The model under review builds one solid part; all positions refer to its coordinate system, in mm. A direction names the side the tool comes from. Give positions to 0.01 mm unless a question says otherwise; leave off trailing zeros. Order: outer loops, then holes, each group sorted by start corner. A loop starts at its lowest first (then second) coordinate and runs counter-clockwise, first axis right, second up. Notation, with made-up numbers: (-23.75, -10) -> (-3.75, -10) arc R21 ccw to (-3.75, 26) -> close; hole circle Ø7 at (-4, 87.25). An arc over 180 degrees is marked (long way). Use one line per item in the form item = value.
```python
from build123d import *

# Parameters (mm, degrees)
SKETCH_W     = 30
SKETCH_H     = 30
PAD_DEPTH    = 2
SKETCH001_W  = 3
SKETCH001_H  = 26
PAD001_DEPTH = 4
SKETCH002_W  = 30
SKETCH002_H  = 2
PAD002_DEPTH = 5
SKETCH003_R  = 1
SKETCH003_W  = 9
SKETCH003_H  = 5
POCKET_DEPTH = 10


with BuildPart() as part:
    # Sketch → Pad (new body)
    with BuildSketch(Plane.XY):
        Rectangle(SKETCH_W, SKETCH_H)
    extrude(amount=PAD_DEPTH)

    # Sketch001 (on Face6 of Pad) → Pad001 (join)
    with BuildSketch(Plane.XY.offset(2)):
        with Locations((-13.5, 0)):
            Rectangle(SKETCH001_W, SKETCH001_H)
        with Locations((13.5, 0)):
            Rectangle(SKETCH001_W, SKETCH001_H)
    extrude(amount=PAD001_DEPTH)

    # Sketch002 (on Face5 of Pad001) → Pad002 (join)
    with BuildSketch(Plane.XY.offset(2)):
        with Locations((0, -14)):
            Rectangle(SKETCH002_W, SKETCH002_H)
        with Locations((0, 14)):
            Rectangle(SKETCH002_W, SKETCH002_H)
    extrude(amount=PAD002_DEPTH)

    # Sketch003 (on Face16 of Pad002) → Pocket (cut)
    with BuildSketch(Plane.XY.offset(7)):
        with Locations((-12.5, 12.5)):
            Circle(SKETCH003_R)
        with Locations((-12.5, -12.5)):
            Circle(SKETCH003_R)
        with Locations((12.5, -12.5)):
            Circle(SKETCH003_R)
        with Locations((12.5, 12.5)):
            Circle(SKETCH003_R)
        with Locations((4.5, -12.5)):
            Rectangle(SKETCH003_W, SKETCH003_H)
    extrude(amount=-POCKET_DEPTH, mode=Mode.SUBTRACT)


solid = part.part
```
1. The part is to be moulded in two halves that separate along X. For faces 4 (the face through (-15, 0, 3)), 5 (the face through (13, 0, 6)), 6 (the face through (9, -14, 3)), say which applies: +X half, -X half, draft (parallel to the pull), parting line (faces both ways), or undercut.
Values:
face_4 = -X half
face_5 = draft
face_6 = undercut
2. Add section D-D on y = -4. Give the boundary of the cut face in (x, z), then the cut area to 3 significant figures.
Values:
outline = (-15, 0) -> (15, 0) -> (15, 6) -> (12, 6) -> (12, 2) -> (-12, 2) -> (-12, 6) -> (-15, 6) -> close
area = 84.0 mm^2
3. Add section B-B on y = 12.5. Give the boundary of the cut face in (x, z), then the cut area to 3 significant figures.
Values:
outline = (-15, 0) -> (-13.5, 0) -> (-13.5, 6) -> (-15, 6) -> close; (-11.5, 0) -> (11.5, 0) -> (11.5, 2) -> (-11.5, 2) -> close; (13.5, 0) -> (15, 0) -> (15, 6) -> (13.5, 6) -> close
area = 64.0 mm^2
4. Tool access review of faces 1 (the face through (14.2, -13, 6.5)), 2 (the face through (0, -14, 3)), 3 (the face through (12, 0, 4)): name each direction out of +Z, -Z, +X, -X, +Y, -Y from which nothing blocks a thin tool from reaching the whole face with its end or side.
Values:
face_1 = +Z, +X, -X
face_2 = +Z, -Z, -Y
face_3 = +Z
5. For pin 1 Ø0.9 at (x, y) = (-13.5, -4.5) entering from +Z; pin 2 Ø1.6 at (x, z) = (2.5, 1) entering from -Y, all flat-tipped, find the tip position at first contact; note any pin that passes through.
Values:
pin_1 = 6
pin_2 = -10
6. Add section C-C on z = 0.75. Give the boundary of the cut face in (x, y).
Values:
outline = (-15, -15) -> (0, -15) -> (0, -10) -> (9, -10) -> (9, -15) -> (15, -15) -> (15, 15) -> (-15, 15) -> close; hole circle Ø2 at (-12.5, -12.5); hole circle Ø2 at (-12.5, 12.5); hole circle Ø2 at (12.5, -12.5); hole circle Ø2 at (12.5, 12.5)
7. Add section A-A on x = -12.5. Give the boundary of the cut face in (y, z), then the cut area to 3 significant figures.
Values:
outline = (-15, 0) -> (-13.5, 0) -> (-13.5, 7) -> (-15, 7) -> close; (-11.5, 0) -> (11.5, 0) -> (11.5, 6) -> (-11.5, 6) -> close; (13.5, 0) -> (15, 0) -> (15, 7) -> (13.5, 7) -> close
area = 159 mm^2
8. For L1, parallel to Y at x = 12.5, z = 2.25; L2, parallel to X at y = 10.5, z = 2.75; L3, parallel to X at y = -12.5, z = 1.75, list the stretches that pass through material, from the lowest coordinate up.
Values:
L1 = -15 to -13.5, -11.5 to 11.5, 13.5 to 15
L2 = -15 to -12, 12 to 15
L3 = -15 to -13.5, -11.5 to 0, 9 to 11.5, 13.5 to 15
